Read the model definition and answer for the solid it produces. Units are mm, in the model's axes. A direction names the side the tool comes from. Coordinates: 2 decimals unless noted, no trailing zeros. Loops run counter-clockwise (first coordinate to the right, second up) from the corner with the lowest first, then second, coordinate; pieces in that order, holes last. Notation, with made-up numbers: (-17, 85.25) -> (35, 85.25) arc R15 ccw to (35, 91.25) -> close; hole circle Ø5 at (85, 3). An arc over 180 degrees is marked (long way). Answer as a JSON object with one key per item and string values. Group by question number.
Q1. The part is cut by section D-D on y = 1.05. Write down the section's boundary in (x, z) (1 decimal), and give its area (3 significant figures).
Q2. Determine the mould class of faces 1 (the flat face through (0, 0, 0)), 2 (the cylindrical face through (-11.414, 0.999, 0.07)), 3 (the cylindrical face through (-16.108, 0.74, -3.577)) for opening direction X: released by +X, released by -X, zero draft, split by the parting line, or undercut.
Q3. The part is cut by section A-A on z = 0. Write down the section's boundary in (x, y).
Q4. The part is cut by section B-B on x = 0. Write down the section's boundary in (y, z), and give its area (3 significant figures).
Q5. The part is cut by section C-C on x = 6. Write down the section's boundary in (y, z), and give its area (3 significant figures).
Q6. This flat-tipped pin is pushed along its axis until it touches: P1, Ø3, axis at x = 13, z = 0, coming from the +Y side. Where does it stop, or does it pass through?
Q7. For faces 4 (the flat face through (14, 0.484, 1)), 5 (the cylindrical face through (0.04, 0.24, 13.89)), determine the directions among +Z, -Z, +X, -X, +Y, -Y from which every point of the face is accessible in a straight line to the end or side of a thin tool.
Q8. Straight lines are drawn through the part: line 1 along Z through (x, y) = (-0.5, 0.1); line 2 along Z through (x, y) = (-13, 1.05); line 3 along X through (y, z) = (1.3, -14). For each, find the intervals that lie inside material, in ascending order. Write a range as [from, to].
from build123d import *

# Parameters (mm, degrees)
SKETCH1_R                                      = 16.5
BOSS_EXTRUDE1_DEPTH                            = 1.5
CBORE_FOR_0_SOCKET_HEAD_CAP_SCREW1_D           = 1.778
CBORE_FOR_0_SOCKET_HEAD_CAP_SCREW1_CBORE_D     = 3.175
CBORE_FOR_0_SOCKET_HEAD_CAP_SCREW1_CBORE_DEPTH = 1.016
CIRPATTERN1_COUNT                              = 4
SKETCH8_R                                      = 0.5
CUT_EXTRUDE1_DEPTH                             = 1.5
SKETCH9_R                                      = 1
CUT_EXTRUDE2_DEPTH                             = 10


with BuildPart() as part:
    # Sketch1 → Boss-Extrude1 (new body)
    with BuildSketch(Plane(origin=(0, 0, 0), x_dir=(1, 0, 0), z_dir=(0, 1, 0))):
        with Locations(Location((0, 0, 0), (0, 0, 270))):
            Circle(SKETCH1_R)
    extrude(amount=BOSS_EXTRUDE1_DEPTH)

    # CBORE for #0 Socket Head Cap Screw1 (through all)
    with Locations(Plane(origin=(0, 1.5, 0), x_dir=(1, 0, 0), z_dir=(0, 1, 0))):
        with Locations((13, 0)):
            cbore_for_0_socket_head_cap_screw1 = CounterBoreHole(CBORE_FOR_0_SOCKET_HEAD_CAP_SCREW1_D / 2, CBORE_FOR_0_SOCKET_HEAD_CAP_SCREW1_CBORE_D / 2, CBORE_FOR_0_SOCKET_HEAD_CAP_SCREW1_CBORE_DEPTH)

    # CirPattern1: CBORE for #0 Socket Head Cap Screw1 ×4 about axis
    cirpattern1_axis = Axis((0, 0, 0), (0, 1, 0))
    for i in range(1, CIRPATTERN1_COUNT):
        add(cbore_for_0_socket_head_cap_screw1.rotate(cirpattern1_axis, i * 360 / CIRPATTERN1_COUNT), mode=Mode.SUBTRACT)

    # Sketch8 → Cut-Extrude1 (cut)
    with BuildSketch(Plane.XZ):
        with Locations(Location((6, 0, 0), (0, 0, 270))):
            Circle(SKETCH8_R)
    extrude(amount=-CUT_EXTRUDE1_DEPTH, mode=Mode.SUBTRACT)

    # Sketch9 → Cut-Extrude2 (cut)
    with BuildSketch(Plane(origin=(0, 1.5, 0), x_dir=(1, 0, 0), z_dir=(0, 1, 0))):
        with Locations(Location((11.591109915, -3.105828541, 0), (0, 0, 270))):
            Circle(SKETCH9_R)
    extrude(amount=-CUT_EXTRUDE2_DEPTH, mode=Mode.SUBTRACT)


solid = part.part
Final values:
{
 "1": {"outline": "circle Ø33 at (0, 0); hole circle Ø3.2 at (-13, 0); hole circle Ø3.2 at (0, -13); hole circle Ø3.2 at (0, 13); hole circle Ø1 at (6, 0); hole circle Ø2 at (11.6, 3.1); hole circle Ø3.2 at (13, 0)", "area": "820 mm2"},
 "2": {"face 1": "zero draft", "face 2": "undercut", "face 3": "split by the parting line"},
 "3": {"outline": "(-16.5, 0) -> (-13.89, 0) -> (-13.89, 0.48) -> (-14.59, 0.48) -> (-14.59, 1.5) -> (-16.5, 1.5) -> close; (-12.11, 0) -> (5.5, 0) -> (5.5, 1.5) -> (-11.41, 1.5) -> (-11.41, 0.48) -> (-12.11, 0.48) -> close; (6.5, 0) -> (12.11, 0) -> (12.11, 0.48) -> (11.41, 0.48) -> (11.41, 1.5) -> (6.5, 1.5) -> close; (13.89, 0) -> (16.5, 0) -> (16.5, 1.5) -> (14.59, 1.5) -> (14.59, 0.48) -> (13.89, 0.48) -> close"},
 "4": {"outline": "(0, -16.5) -> (1.5, -16.5) -> (1.5, -14.59) -> (0.48, -14.59) -> (0.48, -13.89) -> (0, -13.89) -> close; (0, -12.11) -> (0.48, -12.11) -> (0.48, -11.41) -> (1.5, -11.41) -> (1.5, 11.41) -> (0.48, 11.41) -> (0.48, 12.11) -> (0, 12.11) -> close; (0, 13.89) -> (0.48, 13.89) -> (0.48, 14.59) -> (1.5, 14.59) -> (1.5, 16.5) -> (0, 16.5) -> close", "area": "41.3 mm2"},
 "5": {"outline": "(0, -15.37) -> (1.5, -15.37) -> (1.5, -0.5) -> (0, -0.5) -> close; (0, 0.5) -> (1.5, 0.5) -> (1.5, 15.37) -> (0, 15.37) -> close", "area": "44.6 mm2"},
 "6": {"P1": "stops at y = 0.48"},
 "7": {"face 4": "+Y", "face 5": "+Y, -Y"},
 "8": {"line 1": "z = [-16.49, -13.74], [-12.26, 12.26], [13.74, 16.49]", "line 2": "z = [-10.16, -1.59], [1.59, 10.16]", "line 3": "x = [-8.73, -1.23], [1.23, 8.73]"}
}
